Check sheet for the modelled part. Datum: model origin and axes. Units: mm. A direction names the side the tool comes from. Round coordinates to 2 decimals unless told otherwise and drop trailing zeros. Order: outer loops, then holes, each group sorted by start corner. A loop starts at its lowest first (then second) coordinate and runs counter-clockwise, first axis right, second up.
```python
from build123d import *

# Parameters (mm, degrees)
SKETCH1_W           = 66
SKETCH1_H           = 36
BOSS_EXTRUDE1_DEPTH = 3
SKETCH2_W           = 2
SKETCH2_H           = 4
BOSS_EXTRUDE3_DEPTH = 3
SKETCH3_R           = 0.75
CUT_EXTRUDE1_DEPTH  = 40.471508712
SKETCH4_W           = 3
SKETCH4_H           = 15
CUT_EXTRUDE2_DEPTH  = 40.471508712
FILLET2_R           = 2
FILLET3_R           = 1


with BuildPart() as part:
    # Sketch1 → Boss-Extrude1 (new body)
    with BuildSketch(Plane.XY):
        Rectangle(SKETCH1_W, SKETCH1_H)
    extrude(amount=BOSS_EXTRUDE1_DEPTH)

    # Sketch2 → Boss-Extrude3 (add)
    with BuildSketch(Plane.XY.offset(3)):
        with Locations((-34, 16)):
            Rectangle(SKETCH2_W, SKETCH2_H)
        with Locations((-34, -16)):
            Rectangle(SKETCH2_W, SKETCH2_H)
        with Locations((34, 16)):
            Rectangle(SKETCH2_W, SKETCH2_H)
        with Locations((34, -16)):
            Rectangle(SKETCH2_W, SKETCH2_H)
    extrude(amount=-BOSS_EXTRUDE3_DEPTH)

    # Sketch3 → Cut-Extrude1 (cut, through all)
    with BuildSketch(Plane.XY.offset(3)):
        with Locations((-32.5, 16)):
            Circle(SKETCH3_R)
        with Locations(Location((-32.5, -16, 0), (0, 0, 180))):
            Circle(SKETCH3_R)
        with Locations((32.5, -16)):
            Circle(SKETCH3_R)
        with Locations(Location((32.5, 16, 0), (0, 0, 180))):
            Circle(SKETCH3_R)
    extrude(amount=-CUT_EXTRUDE1_DEPTH, mode=Mode.SUBTRACT)

    # Sketch4 → Cut-Extrude2 (cut, through all)
    with BuildSketch(Plane.XY.offset(3)):
        with Locations((-31.5, -1.5)):
            Rectangle(SKETCH4_W, SKETCH4_H)
    extrude(amount=-CUT_EXTRUDE2_DEPTH, mode=Mode.SUBTRACT)

    # Fillet2
    fillet2_edges = [part.edges().sort_by_distance(p)[0] for p in [
        (-33, -9, 1.5),
        (-33, 6, 1.5),
    ]]
    fillet(fillet2_edges, radius=FILLET2_R)

    # Fillet3
    fillet3_edges = [part.edges().sort_by_distance(p)[0] for p in [
        (35, -14, 1.5),
        (33, -14, 1.5),
        (33, 14, 1.5),
        (35, 14, 1.5),
        (35, 18, 1.5),
        (-35, 18, 1.5),
        (-35, 14, 1.5),
        (-33, 14, 1.5),
        (-33, -14, 1.5),
        (-35, -14, 1.5),
    ]]
    fillet(fillet3_edges, radius=FILLET3_R - 0.0001)  # a hair under: the kernel refuses the full size


solid = part.part
```
Item 1: Sectioned sample at C-C (y = -7). Record the cut outline in (x, z).
Answer:
outline: (-30, 0) - (33, 0) - (33, 3) - (-30, 3) - close
Item 2: Scan lines: line 1 along Y through (x, z) = (32.5, 0.7); line 2 along X through (y, z) = (-8.5, 1.9); line 3 along Y through (x, z) = (-32.5, 1.4). Record each from-to range of solid material in increasing order.
Answer:
line 1: y = -18 to -16.75, -15.25 to 15.25, 16.75 to 18
line 2: x = -30 to 33
line 3: y = -18 to -16.75, -15.25 to -9.68, 6.68 to 15.25, 16.75 to 18
Item 3: Release check for a two-part mould opening along Y. For faces 4 (the flat face through (-35, -17, 2)), 5 (the flat face through (0, 18, 2)), 6 (the cylindrical face through (-32.43, 6.6, 1.48)), 7 (the flat face through (0, -18, 1)) record: released by +Y, released by -Y, zero draft, split by the parting line, or undercut.
Answer:
face 4: zero draft
face 5: released by +Y
face 6: undercut
face 7: released by -Y
Item 4: Sectioned sample at A-A (y = -16). Record the cut outline in (x, z), and give its area (3 significant figures).
Answer:
outline: (-35, 0) - (-33.25, 0) - (-33.25, 3) - (-35, 3) - close; (-31.75, 0) - (31.75, 0) - (31.75, 3) - (-31.75, 3) - close; (33.25, 0) - (35, 0) - (35, 3) - (33.25, 3) - close
area: 201 mm2
Item 5: Go/stop test with flat-tipped pins: P1, Ø0.9, axis at y = 11, z = 2, coming from the -X side; P2, Ø1.5, axis at y = 3.5, z = 1, coming from the +X side; P3, Ø1.2, axis at x = 32.5, y = -16, coming from the -Z side; P4, Ø0.9, axis at y = -4, z = 1, coming from the -X side. Record where each tip stops, or that it passes through.
Answer:
P1: stops at x = -33
P2: stops at x = 33
P3: passes through
P4: stops at x = -30
Item 6: Sectioned sample at B-B (z = 1.85). State how many separate pieces and enclosed holes the cut face has, and give its area (3 significant figures).
Answer:
separate pieces: 1
enclosed holes: 4
area: 2,350 mm2
Item 7: Access from +Z, -Z, +X, -X, +Y, -Y to the whole of each face (thin tool, end or side, straight path). Record for faces 1 (the flat face through (35, 16, 2)), 2 (the flat face through (33, 0, 1)), 3 (the flat face through (-33, 10, 1)).
Answer:
face 1: +Z, -Z, +X, +Y, -Y
face 2: +Z, -Z, +X
face 3: +Z, -Z, -X
